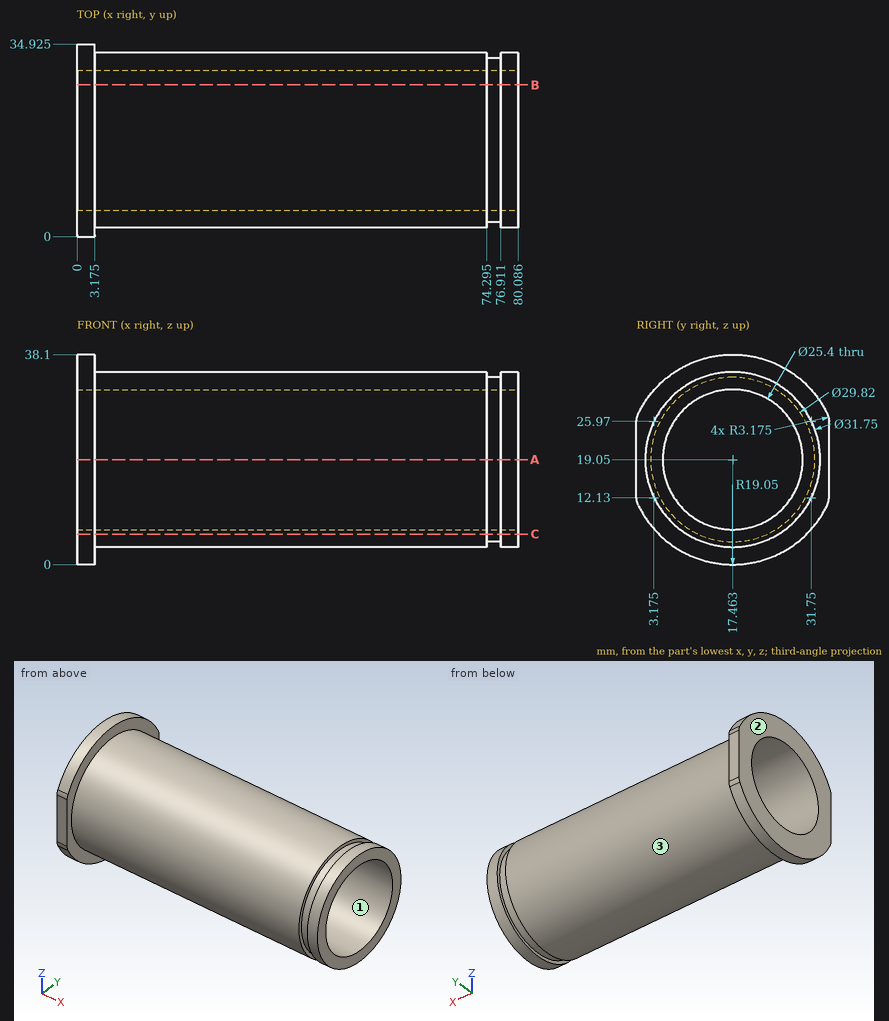
For this review, use the dimensioned drawing (mm, ordinates from the lowest corner) and the shaded views. Give positions to 0.01 mm unless a question says otherwise; leave off trailing zeros. Order: outer loops, then holes, each group sorted by start corner. A loop starts at its lowest first (then second) coordinate and runs counter-clockwise, first axis right, second up.
1) Wall thickness on line 1 (Z direction, x = 56, y = 18) (1 decimal); line 2 (Y direction, x = 54, z = 19.05); line 3 (Z direction, x = 38, y = 13) (1 decimal): over which ranges is each line inside the solid? List them lowest first.
2) The part is to be moulded in two halves that separate along Y. For the marked faces 1, 2 and 3, say which applies: released by +Y, released by -Y, zero draft, split by the parting line, or undercut.
3) Take a section at C-C (z = 5.5). Give the boundary of the cut face in (x, y) (1 decimal).
4) Take a section at B-B (y = 27.5). Give the boundary of the cut face in (x, z) (1 decimal).
5) Take a section at A-A (z = 19.05). Give the boundary of the cut face in (x, y) (1 decimal).
6) Insertion check: pin 1 (2 mm diameter, centred on x = 25, y = 9.5, fed in from +Z); pin 2 (1 mm diameter, centred on x = 68.5, y = 17, fed in from +Z) (1 decimal); pin 3 (8 mm diameter, centred on x = 12, z = 9, fed in from -Y) (1 decimal). Each pin has a flat end and moves straight along its axis. Give the tip position at first contact, or say it passes through.
Derived:
1. line 1: z = 3.2 to 6.4, 31.7 to 34.9
1. line 2: y = 1.59 to 4.76, 30.16 to 33.34
1. line 3: z = 3.8 to 7.2, 30.9 to 34.3
2. face 1: undercut
2. face 2: zero draft
2. face 3: split by the parting line
3. outline: (0, 4.1) - (3.2, 4.1) - (3.2, 9.2) - (74.3, 9.2) - (74.3, 11.2) - (76.9, 11.2) - (76.9, 9.2) - (80.1, 9.2) - (80.1, 25.7) - (76.9, 25.7) - (76.9, 23.7) - (74.3, 23.7) - (74.3, 25.7) - (3.2, 25.7) - (3.2, 30.9) - (0, 30.9) - close
4. outline: (0, 2.9) - (3.2, 2.9) - (3.2, 6.8) - (74.3, 6.8) - (74.3, 8) - (76.9, 8) - (76.9, 6.8) - (80.1, 6.8) - (80.1, 11.3) - (0, 11.3) - close; (0, 26.8) - (80.1, 26.8) - (80.1, 31.3) - (76.9, 31.3) - (76.9, 30.1) - (74.3, 30.1) - (74.3, 31.3) - (3.2, 31.3) - (3.2, 35.2) - (0, 35.2) - close
5. outline: (0, 0) - (3.2, 0) - (3.2, 1.6) - (74.3, 1.6) - (74.3, 2.6) - (76.9, 2.6) - (76.9, 1.6) - (80.1, 1.6) - (80.1, 4.8) - (0, 4.8) - close; (0, 30.2) - (80.1, 30.2) - (80.1, 33.3) - (76.9, 33.3) - (76.9, 32.4) - (74.3, 32.4) - (74.3, 33.3) - (3.2, 33.3) - (3.2, 34.9) - (0, 34.9) - close
6. pin 1: stops at z = 33.32
6. pin 2: stops at z = 34.9
6. pin 3: stops at y = 2.8
